from build123d import *

# Parameters (mm, degrees)
F1_DEPTH = 20
F2_R     = 1.6600926706
F3_R     = 0.231152144


with BuildPart() as f1:
    # F0 (on Front) → F1 (new body)
    with BuildSketch(Plane.XZ):
        with BuildLine():
            ThreePointArc((-44.5080057804, 18.2982461622), (-44.856766986, 8.5238854869), (-41.6028533709, -0.6995524392))
            Line((-41.6028533709, -0.6995524392), (-11.6028533709, -0.6995524392))
            Line((-11.6028533709, -0.6995524392), (-44.5080057804, 18.2982461622))
        make_face()
        with BuildLine():
            ThreePointArc((-37.9288420081, 2.3004475608), (-40.1145449825, 7.0615839207), (-40.1195138693, 12.3004475608))
            Line((-40.1195138693, 12.3004475608), (-22.7990057936, 2.3004475608))
            Line((-22.7990057936, 2.3004475608), (-37.9288420081, 2.3004475608))
        make_face(mode=Mode.SUBTRACT)
    extrude(amount=F1_DEPTH)

    # F2
    f2_edges = [f1.edges().sort_by_distance(p)[0] for p in [
        (-11.602853, -10, -0.699552),
        (-44.508006, -10, 18.298246),
        (-41.602853, -10, -0.699552),
    ]]
    fillet(f2_edges, radius=F2_R)

    # F3
    f3_edges = [f1.edges().sort_by_distance(p)[0] for p in [
        (-22.799006, -10, 2.300448),
        (-37.928842, -10, 2.300448),
        (-40.119514, -10, 12.300448),
    ]]
    fillet(f3_edges, radius=F3_R)


solid = f1.part
Can you work these out from the model? Positions are in its coordinate system, mm. A direction names the side the tool comes from. Give positions to 0.01 mm unless a question says otherwise; leave off trailing zeros. Order: outer loops, then holes, each group sorted by start corner. A loop starts at its lowest first (then second) coordinate and runs counter-clockwise, first axis right, second up. Notation, with made-up numbers: M 50.5,-17 L 85.5,-17 A11 cw 85.5,-3 Z; hole C 0.25,27 d2. An arc over 180 degrees is marked long. One line per question, with ' | ' between items.
Item 1: For faces 1 (the face through (-31.808, -9.86, 7.502)), 2 (the face through (-31, -20, 8)), which set-ups out of +Z, -Z, +X, -X, +Y, -Y let a thin tool reach every point of the face, with its end or its side?
Answer block:
face 1: +Y, -Y | face 2: +Z, -Z, +X, -X, -Y
Item 2: Suppose I cut it at B-B, the plane x = -36.75. Write out the boundary of the cut face in (y, z), then the cut area to 3 significant figures.
Answer block:
outline: M -20,-0.7 L 0,-0.7 L 0,2.3 L -20,2.3 Z; M -20,10.36 L 0,10.36 L 0,13.82 L -20,13.82 Z | area: 129 mm2
Item 3: I'm going to push flat-ended pins straight in: pin 1 Ø4 at (x, y) = (-28.5, -6) entering from +Z; pin 2 Ø2 at (y, z) = (-11.5, 5) entering from +X; pin 3 Ø7 at (x, y) = (-32, -13.5) entering from +Z. Where does each tip first touch, or does it pass through?
Answer block:
pin 1: stops at z = 10.21 | pin 2: stops at x = -19.74 | pin 3: stops at z = 13.1
Item 4: Suppose I cut it at D-D, the plane x = -23. Write out the boundary of the cut face in (y, z).
Answer block:
outline: M -20,-0.7 L 0,-0.7 L 0,5.88 L -20,5.88 Z
Item 5: We'd pull the mould along X, two halves only. Please class faces 3 (the face through (-29, -10, -0.7)), 4 (the face through (-44.046, -10.14, 17.157)), 5 (the face through (-31, -10, 2.3)), 6 (the face through (-40.076, -9.86, 6.892)): released by +X, released by -X, zero draft, split by the parting line, or undercut.
Answer block:
face 3: zero draft | face 4: split by the parting line | face 5: undercut | face 6: undercut
Item 6: Suppose I cut it at A-A, the plane y = -16. Write out the boundary of the cut face in (x, z), then the cut area to 3 significant figures.
Answer block:
outline: M -44.94,15.89 A26.25 ccw -42.09,0.18 A1.66 ccw -40.63,-0.7 L -17.8,-0.7 A1.66 ccw -16.97,2.4 L -42.46,17.12 A1.66 ccw Z; hole M -40.18,11.98 A12.29 ccw -38,2.39 A0.23 ccw -37.81,2.3 L -23.66,2.3 A0.23 ccw -23.55,2.73 L -39.84,12.14 A0.23 ccw Z | area: 217 mm2
Item 7: Suppose I cut it at C-C, the plane z = 8.75. Write out the boundary of the cut face in (x, y), then the cut area to 3 significant figures.
Answer block:
outline: M -44.89,-20 L -40.36,-20 L -40.36,0 L -44.89,0 Z; M -33.97,-20 L -27.97,-20 L -27.97,0 L -33.97,0 Z | area: 211 mm2
Item 8: Please list where these lines run through material, in increasing order: L1, parallel to X at y = -0.75, z = 4.5; L2, parallel to Z at x = -39.25, y = -16; L3, parallel to Z at x = -30.25, y = -16.5.
Answer block:
L1: x = -43.91 to -39.25, -26.61 to -20.61 | L2: z = -0.7 to 4.5, 11.8 to 15.26 | L3: z = -0.7 to 2.3, 6.6 to 10.07
